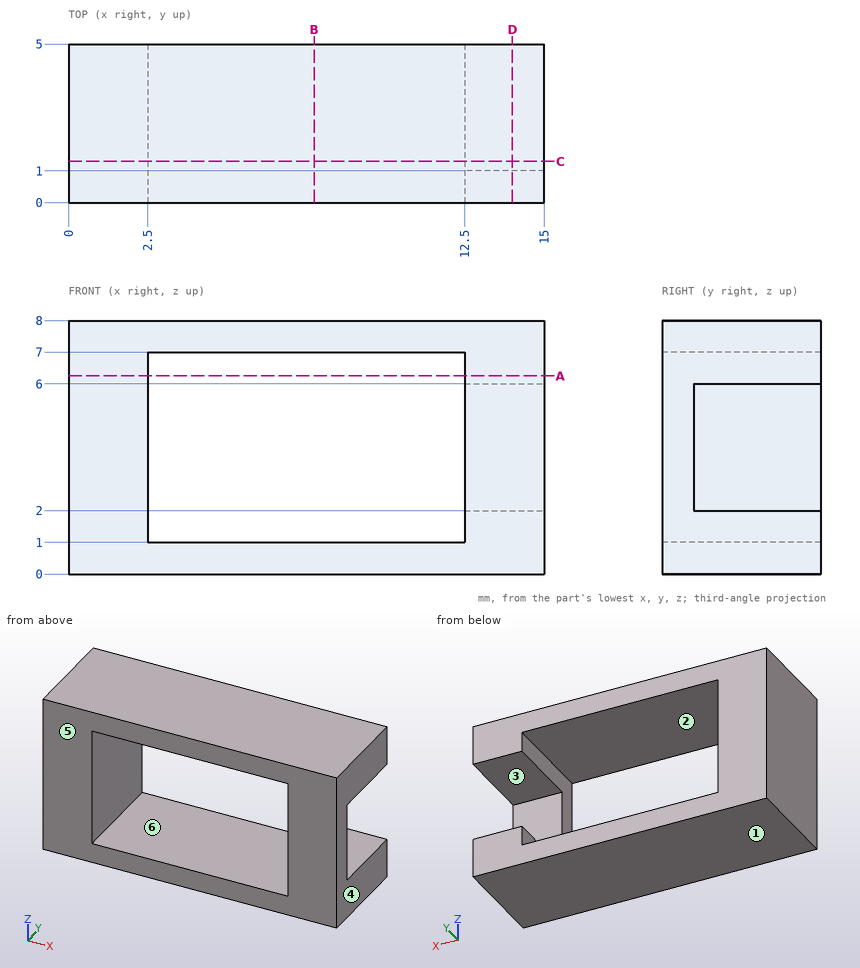
Part print with two shaded views. Sizes in mm from the minimum x, y, z corner. A direction names the side the tool comes from. Round coordinates to 2 decimals unless told otherwise and drop trailing zeros. Order: outer loops, then holes, each group sorted by start corner. A loop starts at its lowest first (then second) coordinate and runs counter-clockwise, first axis right, second up. Notation, with made-up numbers: M 63,-27.5 L 121,-27.5 A18 cw 121,-3.5 Z; hole C 17,-26.5 d4. An arc over 180 degrees is marked long. Use CSV: the item, a comma, the result in double quotes. Start each with the question number.
(1) Drill centre lines: probe 1 along Z at (x, y) = (5, 4.3); probe 2 along X at (y, z) = (3.2, 1.25); probe 3 along X at (y, z) = (4.05, 3). Where is each one in solid material? Low to high.
(2) Cut at D-D on x = 14. List the corners of the cut face in (y, z), then the cut area to 3 significant figures.
(3) Cut at C-C on y = 1.3. List the corners of the cut face in (x, z).
(4) Cut at B-B on x = 7.75. List the corners of the cut face in (y, z), then the cut area to 3 significant figures.
(5) Mould opens along X. For the marked faces 4, 5 and 6 say: +X half, -X half, draft (parallel to the pull), parting line (faces both ways), or undercut.
(6) Tool access for the marked faces 1, 2 and 3: list every direction of +Z, -Z, +X, -X, +Y, -Y with a clear straight run to the whole face (end or side of a thin tool).
(7) Flat gauge pins, fed straight in: P1, Ø3, axis at y = 1.5, z = 6.5, coming from the -X side; P2, Ø0.8, axis at x = 14, z = 5, coming from the +Y side. Where does each tip first touch, or does it go through?
(8) Cut at A-A on z = 6.25. List the corners of the cut face in (x, y), then the cut area to 3 significant figures.
Findings:
1,probe 1,"z = 0 to 1, 7 to 8"
1,probe 2,"x = 0 to 2.5, 12.5 to 15"
1,probe 3,"x = 0 to 2.5"
2,outline,"M 0,0 L 5,0 L 5,2 L 1,2 L 1,6 L 5,6 L 5,8 L 0,8 Z"
2,area,"24.0 mm^2"
3,outline,"M 0,0 L 15,0 L 15,2 L 12.5,2 L 12.5,1 L 2.5,1 L 2.5,7 L 12.5,7 L 12.5,6 L 15,6 L 15,8 L 0,8 Z"
4,outline,"M 0,0 L 5,0 L 5,1 L 0,1 Z; M 0,7 L 5,7 L 5,8 L 0,8 Z"
4,area,"10.0 mm^2"
5,face 4,"+X half"
5,face 5,"draft"
5,face 6,"undercut"
6,face 1,"-Z, +X, -X, +Y, -Y"
6,face 2,"+Y, -Y"
6,face 3,"+X, +Y"
7,P1,"stops at x = 0"
7,P2,"stops at y = 1"
8,outline,"M 0,0 L 2.5,0 L 2.5,5 L 0,5 Z; M 12.5,0 L 15,0 L 15,5 L 12.5,5 Z"
8,area,"25.0 mm^2"
